```python
from build123d import *

# Parameters (mm, degrees)
CUT_EXTRUDE1_DEPTH = 8
CUT_EXTRUDE2_DEPTH = 8
CHAMFER1_SIZE      = 0.5


with BuildPart() as part:
    # Sketch1 → Revolve1 (revolve)
    with BuildSketch(Plane.XY, mode=Mode.PRIVATE) as revolve1_sk:
        Polygon((-6, 2), (-6, 0), (40, 0), (40, 4), (0, 4), (0, 1.6), (-1.2, 1.6), (-1.2, 2), align=None)
    revolve(revolve1_sk.sketch.rotate(Axis((-6, 0, 0), (1, 0, 0)), 270), axis=Axis((-6, 0, 0), (1, 0, 0)))

    # Sketch2 → Cut-Extrude1 (cut)
    with BuildSketch(Plane(origin=(10, 0, 0), x_dir=(0, -1, 0), z_dir=(-1, 0, 0))):
        with BuildLine():
            Line((1.936491673, -3.5), (-1.936491673, -3.5))
            ThreePointArc((-1.936491673, -3.5), (0, -4), (1.936491673, -3.5))
        make_face()
    extrude(amount=-CUT_EXTRUDE1_DEPTH, mode=Mode.SUBTRACT)

    # Sketch3 → Cut-Extrude2 (cut)
    with BuildSketch(Plane(origin=(10, 0, 0), x_dir=(0, -1, 0), z_dir=(-1, 0, 0))):
        with BuildLine():
            Line((-1.936491622, 3.500000028), (1.936491622, 3.500000028))
            ThreePointArc((1.936491622, 3.500000028), (0, 4), (-1.936491622, 3.500000028))
        make_face()
    extrude(amount=-CUT_EXTRUDE2_DEPTH, mode=Mode.SUBTRACT)

    # Chamfer1
    chamfer1_edges = [part.edges().sort_by_distance(p)[0] for p in [
        (-6, 0, 2),
        (0, 0, 4),
        (40, 0, 4),
    ]]
    chamfer(chamfer1_edges, length=CHAMFER1_SIZE)


solid = part.part
```
The model under review builds one solid part; all positions refer to its coordinate system, in mm. A direction names the side the tool comes from. Round coordinates to 2 decimals unless told otherwise and drop trailing zeros. Order: outer loops, then holes, each group sorted by start corner. A loop starts at its lowest first (then second) coordinate and runs counter-clockwise, first axis right, second up.
Item 1: For pin 1 (0.5 mm diameter, centred on y = 0.5, z = 4, fed in from +X); pin 2 (2 mm diameter, centred on x = 25.5, y = -3, fed in from -Z); pin 3 (1 mm diameter, centred on x = 30, z = -0.5, fed in from -Y); pin 4 (1.2 mm diameter, centred on x = 15.5, y = 0, fed in from +Z), all flat-tipped, find the tip position at first contact; note any pin that passes through.
Working result:
pin 1: stops at x = 39.72
pin 2: stops at z = -3.46
pin 3: stops at y = -4
pin 4: stops at z = 3.5
Item 2: To check wall thickness, follow probe 1 along X at (y, z) = (-3.25, -0.5); probe 2 along X at (y, z) = (1.25, 1.5); probe 3 along Z at (x, y) = (38.5, 0.25). State the ranges of each line that lie inside material, in increasing order.
Working result:
probe 1: x = 0 to 40
probe 2: x = -5.55 to -1.2, 0 to 40
probe 3: z = -3.99 to 3.99
Item 3: Add section D-D, the plane x = 36. State the section outline as (y, z) points, and give its area (3 significant figures).
Working result:
outline: circle Ø8 at (0, 0)
area: 50.3 mm2
Item 4: Machinability: for faces 1 (the flat face through (14, 0, -3.5)), 2 (the flat face through (14, 0, 3.5)), 3 (the cylindrical face through (20, 0, 4)), 4 (the cylindrical face through (-3, -2, 0)), 5 (the flat face through (0, -2, -1)), which of the approach directions +Z, -Z, +X, -X, +Y, -Y give a long, thin tool a straight path to every point of the face, cutting with its end or side? Answer none if there is none.
Working result:
face 1: -Z, +Y, -Y
face 2: +Z, +Y, -Y
face 3: +X, -X
face 4: -X
face 5: none
Item 5: Add section B-B, the plane z = 0. State the section outline as (x, y) points.
Working result:
outline: (-6, -1.5) - (-5.5, -2) - (-1.2, -2) - (-1.2, -1.6) - (0, -1.6) - (0, -3.5) - (0.5, -4) - (39.5, -4) - (40, -3.5) - (40, 3.5) - (39.5, 4) - (0.5, 4) - (0, 3.5) - (0, 1.6) - (-1.2, 1.6) - (-1.2, 2) - (-5.5, 2) - (-6, 1.5) - close
Item 6: Add section C-C, the plane x = 11. State the section outline as (y, z) points.
Working result:
outline: (-1.94, -3.5) - (1.94, -3.5) arc R4 ccw to (1.94, 3.5) - (-1.94, 3.5) arc R4 ccw to start
Item 7: Add section A-A, the plane y = 0. State the section outline as (x, z) points.
Working result:
outline: (-6, -1.5) - (-5.5, -2) - (-1.2, -2) - (-1.2, -1.6) - (0, -1.6) - (0, -3.5) - (0.5, -4) - (10, -4) - (10, -3.5) - (18, -3.5) - (18, -4) - (39.5, -4) - (40, -3.5) - (40, 3.5) - (39.5, 4) - (18, 4) - (18, 3.5) - (10, 3.5) - (10, 4) - (0.5, 4) - (0, 3.5) - (0, 1.6) - (-1.2, 1.6) - (-1.2, 2) - (-5.5, 2) - (-6, 1.5) - close
Item 8: Draft analysis for pull direction X (two halves, no side actions). For faces 6 (the flat face through (40, 0, 0)), 7 (the flat face through (-6, 0, 0)), 8 (the cylindrical face through (-0.61, -0.97, 1.27)), state which applies: released by +X, released by -X, zero draft, split by the parting line, or undercut.
Working result:
face 6: released by +X
face 7: released by -X
face 8: undercut
